Drawing for the job (mm, zero at the part's lowest x, y, z). A direction names the side the tool comes from. Coordinates: 2 decimals unless noted, no trailing zeros. Write each loop counter-clockwise with the first axis right and the second up, starting at its lowest first coordinate (ties: lowest second). Pieces come first, ordered by that corner, then holes. Notation, with made-up numbers: M 17.5,-34.5 L 30.5,-34.5 A13 ccw 30.5,-17.5 Z; hole C -30,30 d10. An arc over 180 degrees is marked long. Use a Markdown table: item, result. Add a question column.
Q1. Slice it at A-A on y = 213. Write the cut outline in (x, z).
Q2. Pin check, flat tips, straight feed: pin 1 Ø6 at (y, z) = (216, 602.5) entering from -X; pin 2 Ø3 at (x, y) = (375.5, 184) entering from -Z; pin 3 Ø12 at (x, z) = (353.5, 306.5) entering from -Y. Stop position of each tip, or through.
Q3. Slice it at B-B on x = 458.5. Write the cut outline in (y, z), then the cut area to 3 significant figures.
Q4. Slice it at C-C on z = 94.5. Write the cut outline in (x, y), then the cut area to 3 significant figures.
Q5. Wall check: L1, parallel to X at y = 76.5, z = 614.5; L2, parallel to Y at x = 169, z = 493; L3, parallel to Z at x = 121.5, y = 182. Give the ranges that are in metal, low to high. Write a range as from..to.
Q6. Tool access for the marked faces 5 and 6: list every direction of +Z, -Z, +X, -X, +Y, -Y with a clear straight run to the whole face (end or side of a thin tool).
Q7. Mould opens along X. For the marked faces 1, 2, 3 and 4 say: released by +X, released by -X, zero draft, split by the parting line, or undercut.
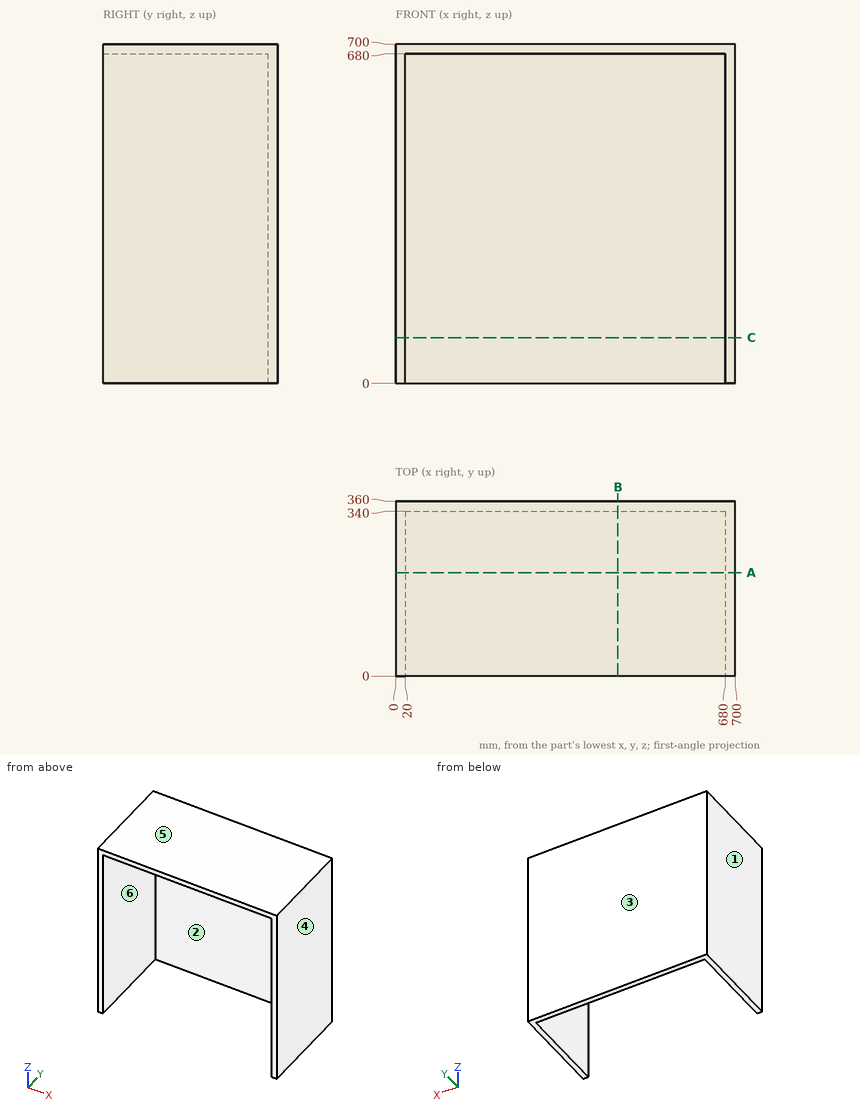
Recorded:
| question | item | result |
|---|---|---|
| 1 | outline | M 0,0 L 20,0 L 20,680 L 680,680 L 680,0 L 700,0 L 700,700 L 0,700 Z |
| 2 | pin 1 | x = 0 |
| 2 | pin 2 | z = 680 |
| 2 | pin 3 | y = 340 |
| 3 | outline | M 0,680 L 340,680 L 340,0 L 360,0 L 360,700 L 0,700 Z |
| 3 | area | 20,800 mm² |
| 4 | outline | M 0,0 L 20,0 L 20,340 L 680,340 L 680,0 L 700,0 L 700,360 L 0,360 Z |
| 4 | area | 27,600 mm² |
| 5 | L1 | 0..20, 680..700 |
| 5 | L2 | 340..360 |
| 5 | L3 | 680..700 |
| 6 | face 5 | +Z, +X, -X, +Y, -Y |
| 6 | face 6 | -Z, -Y |
| 7 | face 1 | released by -X |
| 7 | face 2 | undercut |
| 7 | face 3 | zero draft |
| 7 | face 4 | released by +X |
